Model file for the job. Use its own axes, mm. Face numbers are marked on the shaded views. A direction names the side the tool comes from. Coordinates: 2 decimals unless noted, no trailing zeros. Loops run counter-clockwise (first coordinate to the right, second up) from the corner with the lowest first, then second, coordinate; pieces in that order, holes last. Notation, with made-up numbers: M 54.25,77 L 90.25,77 A31 cw 90.25,107 Z; hole C -12.75,10 d7. An arc over 180 degrees is marked long. Write item = value, one per line. Start each with the question number.
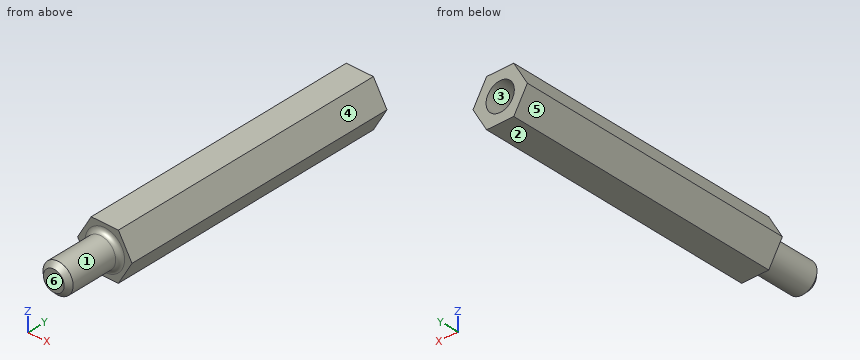
from build123d import *

# Parameters (mm, degrees)
SKETCH1_R           = 1.5
EXTRUDE1_DEPTH      = 30
EXTRUDE2_DEPTH      = 6
EXTRUDE2_DEPTH_BACK = 22
SKETCH2_R           = 1.6
CHAMFER1_SIZE       = 0.5
FILLET1_R           = 0.5
FILLET2_R           = 1


with BuildPart() as part:
    # Sketch1 → Extrude1 (new body)
    with BuildSketch(Plane(origin=(0, 0, 0), x_dir=(1, 0, 0), z_dir=(0, 1, 0))):
        Polygon((-1.443375673, 2.5), (1.443375673, 2.5), (2.886751346, 0), (1.443375673, -2.5), (-1.443375673, -2.5), (-2.886751346, 0), align=None)
        with Locations(Location((0, 0, 0), (0, 0, 270))):
            Circle(SKETCH1_R, mode=Mode.SUBTRACT)
    extrude(amount=EXTRUDE1_DEPTH)

    # Sketch2 → Extrude2 (add, two sides: drawn at the far end of the back side and taken through both)
    with BuildSketch(Plane.XZ.offset(-EXTRUDE2_DEPTH_BACK)):
        with Locations(Location((0, 0, 0), (0, 0, 270))):
            Circle(SKETCH2_R)
    extrude(amount=EXTRUDE2_DEPTH + EXTRUDE2_DEPTH_BACK)

    # Chamfer1
    chamfer1_edges = [part.edges().sort_by_distance(p)[0] for p in [
        (0, -6, 1.6),
    ]]
    chamfer(chamfer1_edges, length=CHAMFER1_SIZE)

    # Fillet1
    fillet1_edges = [part.edges().sort_by_distance(p)[0] for p in [
        (0, 0, 1.6),
    ]]
    fillet(fillet1_edges, radius=FILLET1_R)

    # Fillet2
    fillet2_edges = [part.edges().sort_by_distance(p)[0] for p in [
        (0, 22, -1.5),
    ]]
    fillet(fillet2_edges, radius=FILLET2_R)


solid = part.part
Item 1: Cut at C-C (x = 2.45). Give the cut face in (y, z).
Item 2: 3-axis set-ups, long thin cutter, end or side, ignore diameter. For the marked faces 1 and 2: which of +Z, -Z, +X, -X, +Y, -Y reach the whole face in a straight line?
Item 3: Cut at D-D (x = -2.5). Give the cut face in (y, z).
Item 4: Cut at B-B (y = 5.5). Give the cut face in (x, z), plus the area to 3 significant figures.
Item 5: Probe L1, parallel to Z at x = -0.05, y = 27; L2, parallel to Y at x = 2.4, z = -0.35; L3, parallel to Z at x = 2.05, y = 27. List the from-to ranges inside material, lowest first.
Item 6: Pull direction Z, two halves, no side cores. Call the marked faces 3, 4, 5 and 6: +Z half, -Z half, draft (parallel to the pull), parting line (faces both ways), or undercut.
Item 7: Cut at A-A (y = 28). Give the cut face in (x, z), plus the area to 3 significant figures.
Item 8: Pin check, flat tips, straight feed: pin 1 Ø1.8 at (x, z) = (0, 0) entering from +Y; pin 2 Ø0.8 at (x, z) = (0, 0) entering from +Y; pin 3 Ø1 at (x, z) = (2, -0.5) entering from -Y. Stop position of each tip, or through.
Reported:
q1.outline = M 0,-0.76 L 30,-0.76 L 30,0.76 L 0,0.76 Z
q2.face_1 = -Y
q2.face_2 = -Z, +X, -X, +Y, -Y
q3.outline = M 0,-0.67 L 30,-0.67 L 30,0.67 L 0,0.67 Z
q4.outline = M -2.89,0 L -1.44,-2.5 L 1.44,-2.5 L 2.89,0 L 1.44,2.5 L -1.44,2.5 Z
q4.area = 21.7 mm^2
q5.L1 = -2.5 to -1.5, 1.5 to 2.5
q5.L2 = 0 to 30
q5.L3 = -1.45 to 1.45
q6.face_3 = undercut
q6.face_4 = +Z half
q6.face_5 = -Z half
q6.face_6 = draft
q7.outline = M -2.89,0 L -1.44,-2.5 L 1.44,-2.5 L 2.89,0 L 1.44,2.5 L -1.44,2.5 Z; hole C 0,0 d3
q7.area = 14.6 mm^2
q8.pin_1 = 22.08
q8.pin_2 = 22
q8.pin_3 = -5.54
